Autodesk Inventor part; units mm, degrees
ref_plane "YZ Plane" through (0, 0, 0) normal (1, 0, 0) x (0, 1, 0)
ref_plane "XZ Plane" through (0, 0, 0) normal (0, 1, 0) x (-1, 0, 0)
ref_plane "XY Plane" through (0, 0, 0) normal (0, 0, 1) x (1, 0, 0)
sketch "Sketch1" plane through (0, 0, 0) normal (0, 1, 0) x (-1, 0, 0)
  line L0 (0, 0) -> (450, 0)
  line L1 (450, 0) -> (450, -600)
  line L2 (450, -600) -> (0, -600)
  line L3 (0, -600) -> (0, 0)
  dimension "d0" = 450
  dimension "d1" = 600
extrude "Extrusion1" add sketch "Sketch1" along normal blind 12
sketch "Sketch2" plane through (0, 12, 0) normal (0, 1, 0) x (1, 0, 0)
  line L0 (0, 0) -> (0, 600)
  line L1 (-450, 600) -> (-450, 0)
  line L2 (0, 600) -> (-450, 600)
  line L3 (-450, 600) -> (-450, 0)
  line L4 (-450, 0) -> (0, 0)
  line L5 (0, 0) -> (0, 600)
  line L6 (-438, 588) -> (-12, 588)
  line L7 (-12, 588) -> (-12, 12)
  line L8 (-12, 12) -> (-438, 12)
  line L9 (-438, 12) -> (-438, 588)
  dimension "d4" = 12
extrude "Extrusion2" add sketch "Sketch2" along normal blind 708
sketch "Sketch3" plane through (-450, 0, -600) normal (-1, 0, 0) x (0, 0, 1)
  line L0 (0, 0) -> (40, 0)
  line L1 (40, 0) -> (40, 100)
  line L2 (40, 100) -> (0, 100)
  line L3 (0, 100) -> (0, 0)
  line L4 (600, 0) -> (560, 0)
  line L5 (560, 0) -> (560, 100)
  line L6 (560, 100) -> (600, 100)
  line L7 (600, 100) -> (600, 0)
  line L8 (600, 720) -> (560, 720)
  line L9 (560, 720) -> (560, 620)
  line L10 (560, 620) -> (600, 620)
  line L11 (600, 620) -> (600, 720)
  line L12 (40, 100) -> (560, 100)
  line L13 (560, 100) -> (560, 620)
  line L14 (560, 620) -> (40, 620)
  line L15 (40, 620) -> (40, 100)
  dimension "d7" = 40
  dimension "d8" = 100
  dimension "d9" = 40
  dimension "d10" = 100
  dimension "d11" = 40
  dimension "d12" = 100
extrude "Extrusion3" cut sketch "Sketch3" against normal blind 12 contours L15 L14 L13 L12
sketch "Sketch4" plane through (-12, 12, -588) normal (-1, 0, 0) x (0, 0, 1)
  point P0 (588, -12)
sketch "Sketch5" plane through (-12, 12, -588) normal (-1, 0, 0) x (0, 0, 1)
  line L0 (0, 0) -> (0, 708)
  line L1 (0, 708) -> (0, 688)
  line L2 (576, 0) -> (576, 708)
  line L3 (0, 688) -> (576, 688)
  line L4 (576, 688) -> (576, 676)
  line L5 (576, 676) -> (0, 676)
  line L6 (0, 676) -> (0, 688)
  point P0 (588, -12)
  dimension "d15" = 20
  dimension "d16" = 12
extrude "Extrusion4" add sketch "Sketch5" along normal up to surface (438 mm away)
sketch "Sketch6" plane through (-12, 700, -12) normal (0, 1, 0) x (1, 0, 0)
  line L0 (-426, 576) -> (0, 576)
  line L1 (-213, 576) -> (-213, 0)
  line L2 (0, 0) -> (-426, 0)
  line L3 (-213, 576) -> (-213, 504)
  line L4 (-213, 504) -> (-213, 515)
  line L5 (-213, 515) -> (-113, 515)
  line L6 (-213, 540) -> (-113, 540)
  line L7 (-113, 540) -> (-313, 540)
  line L8 (-313, 540) -> (-313, 518)
  line L9 (-313, 518) -> (-113, 518)
  line L10 (-113, 518) -> (-113, 540)
  line L11 (-213, 529) -> (-338, 529)
  line L12 (-338, 529) -> (-338, 537.5)
  circle A0 centre (-338, 537.5) radius 1.5
  line L13 (-338, 537.5) -> (-338, 520.5)
  circle A1 centre (-338, 520.5) radius 1.5
  circle A2 centre (-88, 537.5) radius 1.5
  circle A3 centre (-88, 520.5) radius 1.5
  line L14 (-213, 518) -> (-213, 374)
  line L15 (-213, 374) -> (-213, 385)
  line L16 (-213, 385) -> (-113, 385)
  line L17 (-113, 385) -> (-313, 385)
  line L18 (-313, 385) -> (-313, 363)
  line L19 (-313, 363) -> (-113, 363)
  line L20 (-113, 363) -> (-113, 385)
  line L21 (-88, 537.5) -> (-88, 520.5)
  line L22 (-113, 374) -> (-88, 374)
  line L23 (-88, 374) -> (-88, 382.5)
  line L24 (-88, 382.5) -> (-88, 365.5)
  circle A4 centre (-88, 382.5) radius 1.5
  circle A5 centre (-88, 365.5) radius 1.5
  circle A6 centre (-338, 382.5) radius 1.5
  circle A7 centre (-338, 365.5) radius 1.5
  line L25 (-213, 288) -> (-149.1067, 288)
  line L26 (-113, 36) -> (-313, 36)
  line L27 (-313, 36) -> (-313, 58)
  line L28 (-313, 58) -> (-113, 58)
  line L29 (-113, 58) -> (-113, 36)
  circle A8 centre (-338, 38.5) radius 1.5
  circle A9 centre (-338, 55.5) radius 1.5
  circle A10 centre (-88, 38.5) radius 1.5
  circle A11 centre (-88, 55.5) radius 1.5
  line L30 (-213, 191) -> (-113, 191)
  line L31 (-113, 191) -> (-313, 191)
  line L32 (-313, 191) -> (-313, 213)
  line L33 (-313, 213) -> (-113, 213)
  line L34 (-113, 213) -> (-113, 191)
  circle A12 centre (-88, 193.5) radius 1.5
  circle A13 centre (-88, 210.5) radius 1.5
  circle A14 centre (-338, 193.5) radius 1.5
  circle A15 centre (-338, 210.5) radius 1.5
  point P0 (12, -12)
  point P1 (-113, 202)
  dimension "d19" = 72
  dimension "d20" = 11
  dimension "d21" = 100
  dimension "d22" = 200
  dimension "d23" = 22
  dimension "d24" = 125
  dimension "d25" = 8.5
  dimension "d26" = 3
  dimension "d27" = 17
  dimension "d28" = 3
  dimension "d29" = 144
  dimension "d30" = 11
  dimension "d31" = 100
  dimension "d32" = 22
  dimension "d33" = 25
  dimension "d34" = 8.5
  dimension "d35" = 17
extrude "Extrusion5" cut sketch "Sketch6" against normal blind 12
sketch "Sketch7" plane through (-12, 700, -12) normal (0, 1, 0) x (1, 0, 0)
  point P0 (12, -12)
sketch "Sketch8" plane through (-12, 700, -12) normal (0, 1, 0) x (1, 0, 0)
  line L0 (-313, 36) -> (-113, 36)
  line L1 (0, 0) -> (-426, 0)
  line L2 (-113, 36) -> (-58, 36)
  line L3 (-58, 36) -> (-58, 0)
  line L4 (-58, 0) -> (-113, 0)
  line L5 (-113, 0) -> (-113, 36)
  line L6 (0, 576) -> (-426, 576)
  line L7 (-58, 0) -> (-113, 0)
  line L8 (-113, 0) -> (-113, 576)
  line L9 (-113, 576) -> (-58, 576)
  line L10 (-58, 576) -> (-58, 0)
  line L11 (-213, 576) -> (-213, 492.9695)
  line L12 (-426, 0) -> (0, 0)
  line L13 (-368, 0) -> (-313, 0)
  line L14 (-426, 576) -> (0, 576)
  line L15 (-313, 0) -> (-313, 576)
  line L16 (-313, 576) -> (-368, 576)
  line L17 (-368, 576) -> (-368, 0)
  line L18 (-313, 518) -> (-113, 518)
  line L19 (-313, 540) -> (-113, 540)
  line L20 (-313, 518) -> (-313, 540)
  line L21 (-113, 213) -> (-313, 213)
  line L22 (-313, 191) -> (-113, 191)
  line L23 (-313, 213) -> (-313, 191)
  line L24 (-313, 202) -> (-313, 152)
  line L25 (-313, 152) -> (-313, 252)
  line L26 (-313, 252) -> (-368, 252)
  line L27 (-313, 152) -> (-368, 152)
  line L28 (-113, 385) -> (-313, 385)
  line L29 (-313, 191) -> (-313, 385)
  line L30 (-313, 288) -> (-113, 288)
  line L31 (-313, 324) -> (-368, 324)
  line L32 (-313, 424) -> (-368, 424)
  line L33 (-113, 252) -> (-58, 252)
  line L34 (-113, 152) -> (-58, 152)
  line L35 (-113, 424) -> (-58, 424)
  line L36 (-113, 324) -> (-58, 324)
  line L37 (-113, 58) -> (-313, 58)
  line L38 (-313, 58) -> (-313, 36)
  line L39 (-313, 47) -> (-313, 97)
  line L40 (-313, 97) -> (-368, 97)
  line L41 (-313, 479) -> (-368, 479)
  line L42 (-113, 97) -> (-58, 97)
  line L43 (-113, 479) -> (-58, 479)
  point P0 (12, -12)
  dimension "d38" = 55
  dimension "d39" = 50
  dimension "d40" = 100
  dimension "d41" = 50
extrude "Extrusion6" cut sketch "Sketch8" against normal blind 6 contours L15 L1 L17 L40 | L8 L42 L10 L2 | L2 L3 L1 L5 | L34 L8 L33 L10 | L17 L26 L15 L27 | L36 L8 L35 L10 | L17 L32 L15 L31 | L43 L8 L6 L10 | L17 L6 L15 L41
properties part number "box"
Build history of the part. All positions in model axes, mm. A direction names the side the tool comes from. Round coordinates to 2 decimals unless told otherwise and drop trailing zeros. Write each loop counter-clockwise with the first axis right and the second up, starting at its lowest first coordinate (ties: lowest second). Pieces come first, ordered by that corner, then holes. Notation, with made-up numbers: (-8.5, 13) - (-0.5, 13) arc R19 cw to (-0.5, 26) - close; hole circle Ø5 at (17, 84.25). An arc over 180 degrees is marked (long way). Write each question's results on one line, items separated by ' | '. Start each with the question number.
Item 1: Drop flat-ended pins along their axis: P1, Ø1, axis at y = 244.5, z = -530.5, coming from the -X side; P2, Ø1, axis at x = -46.5, z = -337.5, coming from the +Y side; P3, Ø1.8, axis at x = -350, z = -394.5, coming from the +Y side. Give the stop position or say it passes through.
Item 2: Saw through at A-A (x = -208.5). Write the cut outline in (y, z).
Item 3: Saw through at B-B (y = 635). Write the cut outline in (x, z).
Item 4: Saw through at D-D (y = 211). Write the cut outline in (x, z).
Item 5: Which spindle directions (+Z, -Z, +X, -X, +Y, -Y) get a long thin tool onto all of the face, cutting with end or side? Do faces 1 (the face through (-226, 720, -590)), 2 (the face through (-228, 345, -588)), 3 (the face through (-353, 694, -540)). Say none if no direction does.
Item 6: Wall check: L1, parallel to X at y = 690.8, z = -549.5; L2, parallel to Z at x = -150.5, y = 610; L3, parallel to Y at x = -405, z = -122. Give the ranges that are in metal, low to high. Write a range as [from, to].
Item 7: Mould opens along Z. For faces 4 (the face through (-222, 345, -12)), 5 (the face through (-228, 355, -600)), 6 (the face through (0, 355, -304)), 7 (the face through (-228, 710, -588)) say: pulls with the +Z half, pulls with the -Z half, needs draft (parallel to the pull), parting line crosses it, or undercut.
Item 8: Saw through at C-C (x = -79). Write the cut outline in (y, z), and give its area (3 significant figures).
Results are:
1) P1: stops at x = -12 | P2: stops at y = 700 | P3: stops at y = 12
2) outline: (0, -600) - (720, -600) - (720, -588) - (700, -588) - (700, -552) - (688, -552) - (688, -588) - (12, -588) - (12, -12) - (688, -12) - (688, -48) - (700, -48) - (700, -12) - (720, -12) - (720, 0) - (0, 0) - close; (688, -530) - (700, -530) - (700, -397) - (688, -397) - close; (688, -375) - (700, -375) - (700, -225) - (688, -225) - close; (688, -203) - (700, -203) - (700, -70) - (688, -70) - close
3) outline: (-450, -600) - (0, -600) - (0, 0) - (-450, 0) - close; hole (-438, -588) - (-12, -588) - (-12, -12) - (-438, -12) - close
4) outline: (-450, -600) - (0, -600) - (0, 0) - (-450, 0) - (-450, -40) - (-438, -40) - (-438, -12) - (-12, -12) - (-12, -588) - (-438, -588) - (-438, -560) - (-450, -560) - close
5) face 1: +Z, -Z, +X, -X, +Y | face 2: none | face 3: +Y
6) L1: x = [-450, -351.5], [-348.5, -325], [-125, -101.5], [-98.5, 0] | L2: z = [-600, -588], [-12, 0] | L3: y = [0, 12], [688, 700]
7) face 4: undercut | face 5: pulls with the -Z half | face 6: needs draft | face 7: undercut
8) outline: (0, -600) - (720, -600) - (720, -588) - (694, -588) - (694, -491) - (700, -491) - (700, -436) - (694, -436) - (694, -336) - (700, -336) - (700, -264) - (694, -264) - (694, -164) - (700, -164) - (700, -109) - (694, -109) - (694, -12) - (720, -12) - (720, 0) - (0, 0) - close; hole (12, -588) - (688, -588) - (688, -12) - (12, -12) - close | area: 28,700 mm²
